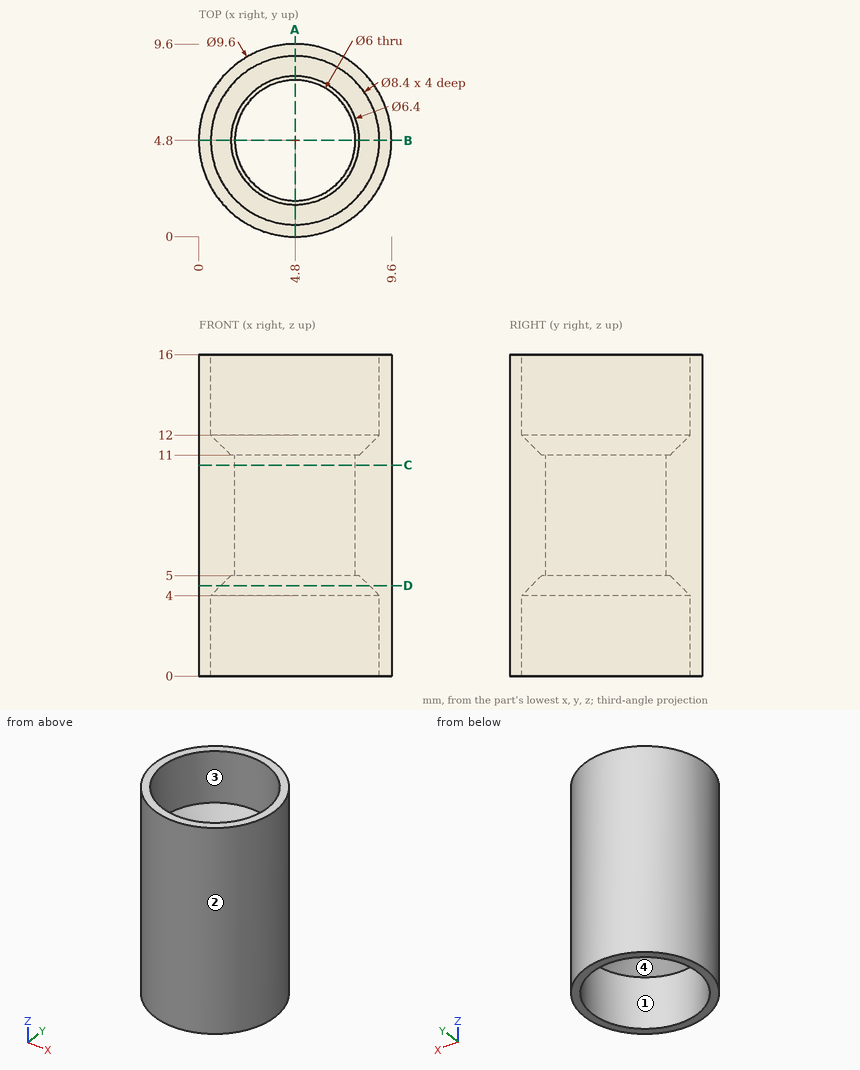
For this review, use the dimensioned drawing (mm, ordinates from the lowest corner) and the shaded views. A direction names the side the tool comes from. Coordinates: 2 decimals unless noted, no trailing zeros. Write each loop counter-clockwise with the first axis right and the second up, starting at its lowest first coordinate (ties: lowest second). Pieces come first, ordered by that corner, then holes. Notation, with made-up numbers: (54, -1.5) - (59, -1.5) arc R16 cw to (59, 26.5) - close; hole circle Ø9 at (-34.5, -23). An arc over 180 degrees is marked (long way). One line per item, written item: value.
1) For the marked faces 3 and 4, list the 3-axis set-ups (+Z, -Z, +X, -X, +Y, -Y) from which the entire face can be reached by the end or side of a thin tool; tool diameter is ignored.
Answer sheet:
face 3: +Z
face 4: -Z
2) Add section C-C (z = 10.5). State the section outline as (x, y) points.
Answer sheet:
outline: circle Ø9.6 at (4.8, 4.8); hole circle Ø6 at (4.8, 4.8)
3) To check wall thickness, follow probe 1 along Y at (x, z) = (4.8, 1.85); probe 2 along X at (y, z) = (7.5, 15); probe 3 along X at (y, z) = (2, 13). State the ranges of each line that lie inside material, in increasing order.
Answer sheet:
probe 1: y = 0 to 0.6, 9 to 9.6
probe 2: x = 0.83 to 1.58, 8.02 to 8.77
probe 3: x = 0.9 to 1.67, 7.93 to 8.7
4) Add section A-A (x = 4.8). State the section outline as (y, z) points.
Answer sheet:
outline: (0, 0) - (0.6, 0) - (0.6, 4) - (1.6, 5) - (1.8, 5) - (1.8, 11) - (1.6, 11) - (0.6, 12) - (0.6, 16) - (0, 16) - close; (7.8, 5) - (8, 5) - (9, 4) - (9, 0) - (9.6, 0) - (9.6, 16) - (9, 16) - (9, 12) - (8, 11) - (7.8, 11) - close
5) Insertion check: pin 1 (3 mm diameter, centred on x = 5, y = 5, fed in from -Z); pin 2 (3 mm diameter, centred on x = 1, z = 6, fed in from -Y); pin 3 (4 mm diameter, centred on y = 1.5, z = 10, fed in from -X). Each pin has a flat end and moves straight along its axis. Give the tip position at first contact, or say it passes through.
Answer sheet:
pin 1: passes through
pin 2: stops at y = 0.59
pin 3: stops at x = 0.18
6) Mouldability with a two-part tool opening along Y and no side actions: class the marked faces 1 and 2 as +Y half, -Y half, draft (parallel to the pull), parting line (faces both ways), or undercut.
Answer sheet:
face 1: undercut
face 2: parting line
7) Add section D-D (z = 4.5). State the section outline as (x, y) points, plus the area to 3 significant figures.
Answer sheet:
outline: circle Ø9.6 at (4.8, 4.8); hole circle Ø7.4 at (4.8, 4.8)
area: 29.4 mm2
